The listing builds one solid part. Answer for the finished solid, in the listing's coordinates (mm). A direction names the side the tool comes from. Give positions to 0.01 mm unless a question says otherwise; leave off trailing zeros. Order: outer loops, then holes, each group sorted by start corner. A loop starts at its lowest first (then second) coordinate and runs counter-clockwise, first axis right, second up. Notation, with made-up numbers: (-38.5, 43) - (-14.5, 43) arc R26 ccw to (-14.5, 59) - close; hole circle Ø11 at (13, 74). An arc over 180 degrees is marked (long way). Use a Markdown table: item, result. Add a question column.
1) Flat-ended cylindrical pins translate along their axes: pin 1 (10 mm diameter, centred on x = -43.5, z = 5.5, fed in from -Y); pin 2 (6 mm diameter, centred on y = 46.5, z = 8.5, fed in from +X); pin 3 (5 mm diameter, centred on x = -55.5, z = 10.5, fed in from +Y); pin 4 (10 mm diameter, centred on x = -69.5, y = 79, fed in from -Z). Find the tip coordinate at first contact, or state that the pin passes through.
2) Find section A-A, the plane z = 2.75. Determine the outline of the cut face in (x, y), plus the area to 3 significant figures.
3) The mould has two halves that part along X. Classify faces 1 (the face through (-84.8, -14, 10.1)), 2 (the face through (-63, 83, 0)), 3 (the face through (-29, 28, 15.24)): released by +X, released by -X, zero draft, split by the parting line, or undercut.
4) Find section B-B, the plane z = 12. Determine the outline of the cut face in (x, y), plus the area to 3 significant figures.
5) For faces 4 (the face through (-29, 30, 20.32)), 5 (the face through (30.27, 53.63, 7.51)), determine the directions among +Z, -Z, +X, -X, +Y, -Y from which every point of the face is accessible in a straight line to the end or side of a thin tool.
6) Straight lines are drawn through the part: line 1 (Y direction, x = -28, z = 7); line 2 (Y direction, x = -22.5, z = 5.5); line 3 (X direction, y = -15.5, z = 6.25). For each, find the intervals that lie inside material, in ascending order.
from build123d import *

# Parameters (mm, degrees)
F0_R     = 71.12
F1_DEPTH = 20.32
F2_R     = 63.5
F3_DEPTH = 15.24
F4_R     = 5.08


with BuildPart() as f1:
    # F0 (on Top) → F1 (new body)
    with BuildSketch(Plane.XY):
        with Locations((-28.390646, 29.312419)):
            Circle(F0_R)
    extrude(amount=F1_DEPTH)

    # F2 (on face) → F3 (cut)
    with BuildSketch(Plane(origin=(0, 0, 0), x_dir=(1, 0, 0), z_dir=(0, 0, -1))):
        with Locations((-28.390646, -29.312419)):
            Circle(F2_R)
    extrude(amount=-F3_DEPTH, mode=Mode.SUBTRACT)

    # F4
    f4_edges = [f1.edges().sort_by_distance(p)[0] for p in [
        (-99.510646, 29.312419, 20.32),
        (-99.510646, 29.312419, 0),
    ]]
    fillet(f4_edges, radius=F4_R)


solid = f1.part
The answers:
| question | item | result |
|---|---|---|
| 1 | pin 1 | y = -41.09 |
| 1 | pin 2 | x = 41.3 |
| 1 | pin 3 | y = 96.04 |
| 1 | pin 4 | z = 0 |
| 2 | outline | circle Ø141.11 at (-28.39, 29.31); hole circle Ø127 at (-28.39, 29.31) |
| 2 | area | 2,970 mm2 |
| 3 | face 1 | split by the parting line |
| 3 | face 2 | zero draft |
| 3 | face 3 | undercut |
| 4 | outline | circle Ø142.24 at (-28.39, 29.31); hole circle Ø127 at (-28.39, 29.31) |
| 4 | area | 3,220 mm2 |
| 5 | face 4 | +Z, +X, -X, +Y, -Y |
| 5 | face 5 | -Z |
| 6 | line 1 | -41.81 to -34.19, 92.81 to 100.43 |
| 6 | line 2 | -41.56 to -33.91, 92.54 to 100.19 |
| 6 | line 3 | -83.62 to -73.38, 16.6 to 26.84 |
